from build123d import *

# Parameters (mm, degrees)
P_IDAT_VYSUNUT_M1_DEPTH = 45
SKICA3_W                = 12.4
SKICA3_H                = 5
P_IDAT_VYSUNUT_M2_DEPTH = 2


with BuildPart() as part:
    # Skica1 → Přidat vysunutím1 (new body)
    with BuildSketch(Plane(origin=(0, 0, 0), x_dir=(1, 0, 0), z_dir=(0, 1, 0))):
        Polygon((-5, 0), (5, 0), (5, 1.6), (4, 2.6), (4, 3), (5, 3), (5, 3.6), (6.2, 3.6), (6.2, -1), (-6.2, -1), (-6.2, 3.6), (-5, 3.6), (-5, 3), (-4, 3), (-4, 2.6), (-5, 1.6), align=None)
    extrude(amount=P_IDAT_VYSUNUT_M1_DEPTH)

    # Skica3 → Přidat vysunutím2 (add)
    with BuildSketch(Plane.XY.offset(1)):
        with Locations((0, 42.5)):
            Rectangle(SKICA3_W, SKICA3_H)
        with Locations((0, 2.5)):
            Rectangle(SKICA3_W, SKICA3_H)
    extrude(amount=P_IDAT_VYSUNUT_M2_DEPTH)


solid = part.part
The listing builds one solid part. Answer for the finished solid, in the listing's coordinates (mm). A direction names the side the tool comes from. Round coordinates to 2 decimals unless told otherwise and drop trailing zeros. Order: outer loops, then holes, each group sorted by start corner. A loop starts at its lowest first (then second) coordinate and runs counter-clockwise, first axis right, second up. Notation, with made-up numbers: (-1.75, -32.5) -> (21.25, -32.5) arc R19 cw to (21.25, -10.5) -> close; hole circle Ø5 at (-9, -17.75). An arc over 180 degrees is marked (long way). Put each result on its own line as item: value.
Q1. Determine the mould class of faces 1 (the flat face through (-6.2, 22, -1)), 2 (the flat face through (0, 22, 0)), 3 (the flat face through (-5, 22, -1)), 4 (the flat face through (-6, 22, -3.6)) for opening direction X: pulls with the +X half, pulls with the -X half, needs draft (parallel to the pull), parting line crosses it, or undercut.
Results list:
face 1: pulls with the -X half
face 2: undercut
face 3: undercut
face 4: needs draft
Q2. Section B-B, the plane z = 1.5 is taken. Write down the section's boundary in (x, y).
Results list:
outline: (-6.2, 0) -> (6.2, 0) -> (6.2, 5) -> (-6.2, 5) -> close; (-6.2, 40) -> (6.2, 40) -> (6.2, 45) -> (-6.2, 45) -> close
Q3. Each of these flat-tipped pins is pushed along its axis until it touches: P1, Ø6, axis at x = -3, y = 23.5, coming from the +Z side; P2, Ø1, axis at x = 1, z = 2, coming from the -Y side; P3, Ø3, axis at x = 0, y = 16, coming from the -Z side; P4, Ø0.5, axis at x = -4.5, y = 26, coming from the -Z side. Where does it stop, or does it pass through?
Results list:
P1: z = 1
P2: y = 0
P3: z = 0
P4: z = -3
Q4. Which of the six approach directions +Z, -Z, +X, -X, +Y, -Y give full straight-line access (tool end or side, diameter ignored) to faces 5 (the flat face through (0, 40, 2)), 6 (the flat face through (5, 22, -1)), 7 (the flat face through (4.5, 22.2, -3))?
Results list:
face 5: +Z, +X, -X
face 6: +Y, -Y
face 7: -Z, +Y, -Y
Q5. Section D-D, the plane y = 34 is taken. Write down the section's boundary in (x, z), and give its area (3 significant figures).
Results list:
outline: (-6.2, -3.6) -> (-5, -3.6) -> (-5, -3) -> (-4, -3) -> (-4, -2.6) -> (-5, -1.6) -> (-5, 0) -> (5, 0) -> (5, -1.6) -> (4, -2.6) -> (4, -3) -> (5, -3) -> (5, -3.6) -> (6.2, -3.6) -> (6.2, 1) -> (-6.2, 1) -> close
area: 22.8 mm^2
Q6. Section C-C, the plane x = 2.5 is taken. Write down the section's boundary in (y, z), and give its area (3 significant figures).
Results list:
outline: (0, 0) -> (45, 0) -> (45, 3) -> (40, 3) -> (40, 1) -> (5, 1) -> (5, 3) -> (0, 3) -> close
area: 65.0 mm^2
Q7. Consider line 1 along Y through (x, z) = (-5.25, 1.5); line 2 along X through (y, z) = (7, -1); line 3 along Z through (x, y) = (0.5, 26). Determine where each line is inside the solid, lowest interval first.
Results list:
line 1: 0 to 5, 40 to 45
line 2: -6.2 to -5, 5 to 6.2
line 3: 0 to 1
Q8. Section A-A, the plane x = -4.5 is taken. Write down the section's boundary in (y, z).
Results list:
outline: (0, -3) -> (45, -3) -> (45, -2.1) -> (0, -2.1) -> close; (0, 0) -> (45, 0) -> (45, 3) -> (40, 3) -> (40, 1) -> (5, 1) -> (5, 3) -> (0, 3) -> close
